Input: dimensioned drawing with shaded views. Units: mm. Origin: part minimum x, y, z. Coordinates: 2 decimals unless noted, no trailing zeros. Order: outer loops, then holes, each group sorted by start corner. A loop starts at its lowest first (then second) coordinate and runs counter-clockwise, first axis right, second up. Notation, with made-up numbers: (3, 57) - (16, 57) arc R13 ccw to (16, 74) - close; hole circle Ø8 at (82.5, 24). An arc over 180 degrees is marked (long way). Use one line per item in the form item = value. Start each with the question number.
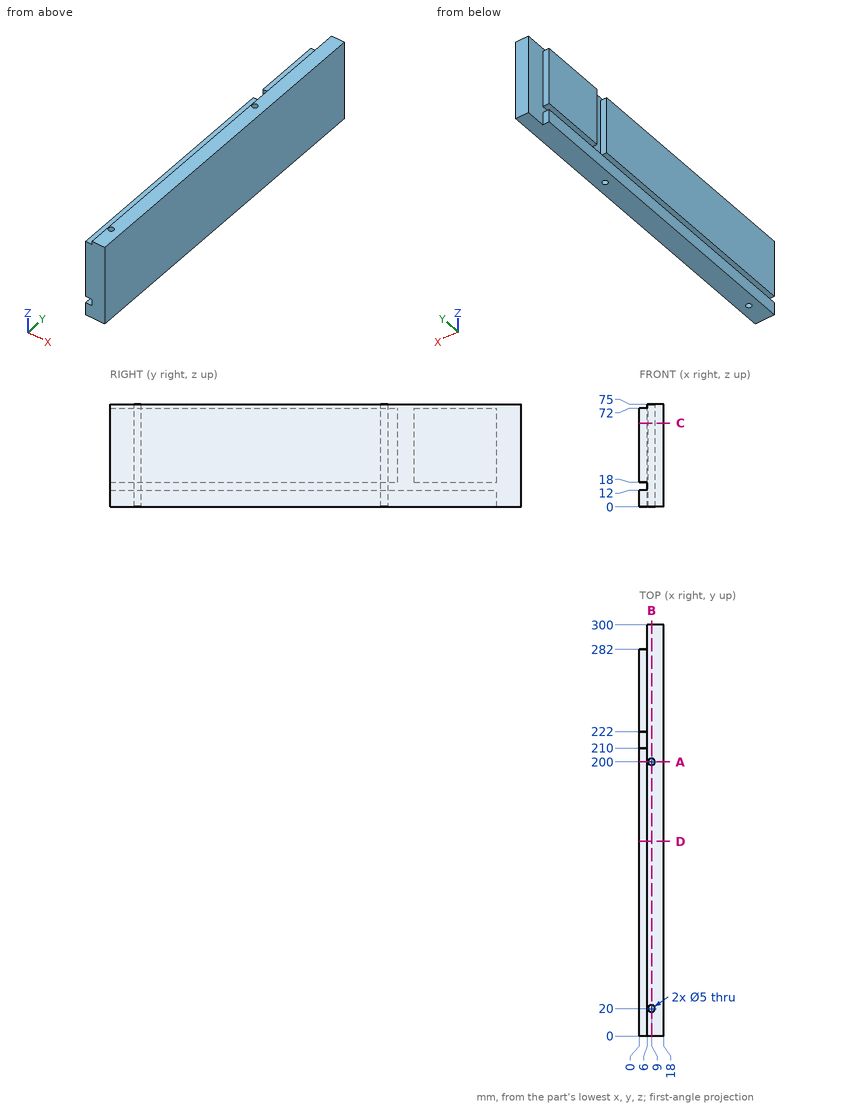
(1) Material intervals for L1, parallel to Y at x = 9, z = 54; L2, parallel to Y at x = 10, z = 44; L3, parallel to X at y = 200, z = 32, sorted ascending. Write a range as from..to.
(2) Cut plane B-B on x = 9. Return the cut outline in (y, z), plus the area to 4 significant figures.
(3) Cut plane C-C on z = 61. Return the cut outline in (x, y).
(4) Cut plane A-A on y = 200. Return the cut outline in (x, z).
(5) Cut plane D-D on y = 142. Return the cut outline in (x, z).
(6) Contact query for flat-ended pins moving along their axis: pin 1 Ø3 at (x, z) = (4, 42.5) entering from +Y; pin 2 Ø6.5 at (x, y) = (2, 238) entering from +Z. Output: stop coordinate, or through.
Check sheet entries:
q1.L1 = 0..17.5, 22.5..197.5, 202.5..300
q1.L2 = 0..17.71, 22.29..197.71, 202.29..300
q1.L3 = 0..6.5, 11.5..18
q2.outline = (0, 0) - (17.5, 0) - (17.5, 75) - (0, 75) - close; (22.5, 0) - (197.5, 0) - (197.5, 75) - (22.5, 75) - close; (202.5, 0) - (300, 0) - (300, 75) - (202.5, 75) - close
q2.area = 21,750 mm^2
q3.outline = (0, 0) - (18, 0) - (18, 300) - (6, 300) - (6, 282) - (0, 282) - (0, 222) - (6, 222) - (6, 210) - (0, 210) - close; hole circle Ø5 at (9, 20); hole circle Ø5 at (9, 200)
q4.outline = (0, 0) - (6.5, 0) - (6.5, 75) - (6, 75) - (6, 72) - (0, 72) - (0, 18) - (6, 18) - (6, 12) - (0, 12) - close; (11.5, 0) - (18, 0) - (18, 75) - (11.5, 75) - close
q5.outline = (0, 0) - (18, 0) - (18, 75) - (6, 75) - (6, 72) - (0, 72) - (0, 18) - (6, 18) - (6, 12) - (0, 12) - close
q6.pin_1 = 282
q6.pin_2 = 72
